Check sheet for the modelled part. Datum: model origin and axes. Units: mm. A direction names the side the tool comes from. Coordinates: 2 decimals unless noted, no trailing zeros. Order: outer loops, then holes, each group sorted by start corner. A loop starts at its lowest first (then second) coordinate and runs counter-clockwise, first axis right, second up.
from build123d import *

# Parameters (mm, degrees)
CROQUIS1_R              = 2.95
SALIENTE_EXTRUIR1_DEPTH = 10
REDONDEO1_R             = 2.5
CROQUIS2_R              = 3.1
SALIENTE_EXTRUIR2_DEPTH = 0.6
CROQUIS5_W              = 0.9
CROQUIS5_H              = 3.9
SALIENTE_EXTRUIR4_DEPTH = 27
CROQUIS8_W              = 0.9
CROQUIS8_H              = 3.9
SALIENTE_EXTRUIR5_DEPTH = 2


with BuildPart() as part:
    # Croquis1 → Saliente-Extruir1 (new body)
    with BuildSketch(Plane(origin=(0, 0, 0), x_dir=(0, 0, -1), z_dir=(1, 0, 0))):
        Circle(CROQUIS1_R)
    extrude(amount=SALIENTE_EXTRUIR1_DEPTH)

    # Redondeo1
    redondeo1_edges = [part.edges().sort_by_distance(p)[0] for p in [
        (10, 0, 2.95),
    ]]
    fillet(redondeo1_edges, radius=REDONDEO1_R)

    # Croquis2 → Saliente-Extruir2 (add)
    with BuildSketch(Plane.ZY):
        Circle(CROQUIS2_R)
    extrude(amount=SALIENTE_EXTRUIR2_DEPTH)

    # Croquis5 → Saliente-Extruir4 (add)
    with BuildSketch(Plane.XY.offset(2.949336532)):
        with Locations((2.848707903, 0)):
            Rectangle(CROQUIS5_W, CROQUIS5_H)
    extrude(amount=SALIENTE_EXTRUIR4_DEPTH)

    # Croquis8 → Saliente-Extruir5 (add)
    with BuildSketch(Plane(origin=(0, 0, 2.949336532), x_dir=(-1, 0, 0), z_dir=(0, 0, -1))):
        with Locations((-2.848707903, 0)):
            Rectangle(CROQUIS8_W, CROQUIS8_H)
    extrude(amount=SALIENTE_EXTRUIR5_DEPTH)


solid = part.part
(1) Thickness scan on probe 1 along X at (y, z) = (-0.5, 20.5); probe 2 along Y at (x, z) = (7.25, 0); probe 3 along Z at (x, y) = (0.5, 1). Record the ranges inside material, lowest first.
Filled in:
probe 1: x = 2.4 to 3.3
probe 2: y = -2.95 to 2.95
probe 3: z = -2.78 to 2.78
(2) Cross-section at A-A (x = 1). Enter the section's corners in (y, z).
Filled in:
outline: circle Ø5.9 at (0, 0)
(3) Release check for a two-part mould opening along X. For faces 4 (the cylindrical face through (-0.3, -2.75, 1.43)), 5 (the flat face through (-0.6, 0, 0)), 6 (the flat face through (3.299, 0, 16)) record: +X half, -X half, draft (parallel to the pull), parting line (faces both ways), or undercut.
Filled in:
face 4: draft
face 5: -X half
face 6: +X half
(4) Go/stop test with flat-tipped pins: P1, Ø2, axis at y = 0, z = 22, coming from the +X side; P2, Ø0.5, axis at x = 3, z = 9.5, coming from the +Y side; P3, Ø1, axis at y = -2.5, z = 24, coming from the -X side; P4, Ø0.5, axis at x = 3, z = 9.5, coming from the -Y side. Record where each tip stops, or that it passes through.
Filled in:
P1: stops at x = 3.3
P2: stops at y = 1.95
P3: passes through
P4: stops at y = -1.95
(5) Tool access check on faces 1 (the flat face through (3, -1.95, 16)), 2 (the flat face through (3, 1.95, 16)), 3 (the flat face through (3, 0, 29.949)). Record the directions out of +Z, -Z, +X, -X, +Y, -Y that give a thin tool (end or side, any length) a straight path to the whole face; none if there is none.
Filled in:
face 1: +Z, +X, -X, -Y
face 2: +Z, +X, -X, +Y
face 3: +Z, +X, -X, +Y, -Y
(6) Cross-section at B-B (z = 28.5). Enter the section's corners in (x, y).
Filled in:
outline: (2.4, -1.95) - (3.3, -1.95) - (3.3, 1.95) - (2.4, 1.95) - close
